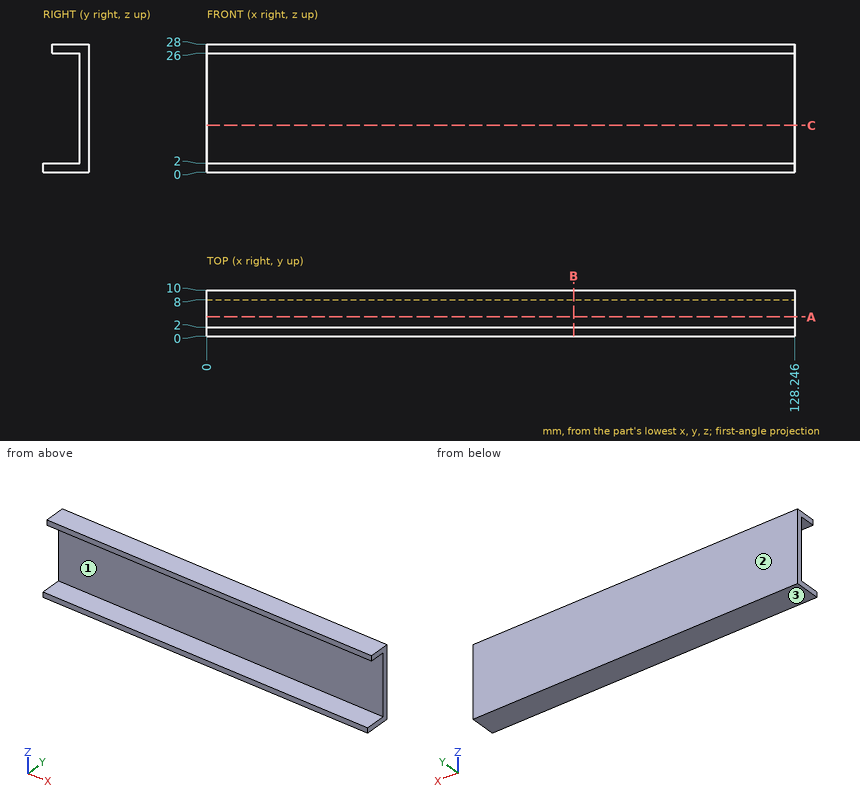
Job drawing, mm, ordinate dimensions from the low corner. One solid piece. Round coordinates to 2 decimals unless told otherwise and drop trailing zeros. Order: outer loops, then holes, each group sorted by start corner. A loop starts at its lowest first (then second) coordinate and runs counter-clockwise, first axis right, second up. Notation, with made-up numbers: M 85.5,82 L 105.5,82 A17 ccw 105.5,97 Z; hole C 54.25,-11 d5. An arc over 180 degrees is marked long. Write each question's results on one line, items separated by ' | '. Start each with the question number.
(1) Two-plate mould, pull along Z, no slides. Class the marked faces 1, 2 and 3: pulls with the +Z half, pulls with the -Z half, needs draft (parallel to the pull), parting line crosses it, or undercut.
(2) Drop flat-ended pins along their axis: pin 1 (1.6 mm diameter, centred on x = 94, z = 27, fed in from -Y); pin 2 (4 mm diameter, centred on x = 21.5, z = 18, fed in from -Y). Give the stop position or say it passes through.
(3) Saw through at B-B, the plane x = 80. Give the cut face in (y, z).
(4) Saw through at C-C, the plane z = 10.25. Give the cut face in (x, y), then the cut area to 4 significant figures.
(5) Probe probe 1 along Z at (x, y) = (33, 7.75); probe 2 along Y at (x, z) = (30.5, 3); probe 3 along Y at (x, z) = (88.5, 26.75). List the from-to ranges inside material, lowest first. Write a range as from..to.
(6) Saw through at A-A, the plane y = 4.25. Give the cut face in (x, z).
Established:
1) face 1: undercut | face 2: needs draft | face 3: pulls with the -Z half
2) pin 1: stops at y = 2 | pin 2: stops at y = 8
3) outline: M 0,0 L 10,0 L 10,28 L 2,28 L 2,26 L 8,26 L 8,2 L 0,2 Z
4) outline: M 0,8 L 128.25,8 L 128.25,10 L 0,10 Z | area: 256.5 mm^2
5) probe 1: z = 0..2, 26..28 | probe 2: y = 8..10 | probe 3: y = 2..10
6) outline: M 0,0 L 128.25,0 L 128.25,2 L 0,2 Z; M 0,26 L 128.25,26 L 128.25,28 L 0,28 Z
